```python
from build123d import *

# Parameters (mm, degrees)
F1_DEPTH = 18.1


with BuildPart() as f1:
    # F0 (on Top) → F1 (new body)
    with BuildSketch(Plane.XY):
        with BuildLine():
            ThreePointArc((24.797365, -3.176582), (24.94929, -1.591519), (25, 0))
            ThreePointArc((25, 0), (24.950482, 1.57272), (24.802124, 3.13921))
            ThreePointArc((24.802124, 3.13921), (24.5233, 4.858782), (24.125403, 6.554762))
            ThreePointArc((24.125403, 6.554762), (23.10419, 9.54968), (21.712851, 12.391614))
            ThreePointArc((21.712851, 12.391614), (20.7972, 13.87359), (19.780568, 15.288203))
            ThreePointArc((19.780568, 15.288203), (17.690984, 17.664345), (15.317994, 19.757507))
            ThreePointArc((15.317994, 19.757507), (13.904914, 20.776269), (12.42432, 21.694153))
            ThreePointArc((12.42432, 21.694153), (9.584486, 23.089773), (6.59111, 24.115498))
            ThreePointArc((6.59111, 24.115498), (4.895732, 24.51595), (3.176582, 24.797365))
            ThreePointArc((3.176582, 24.797365), (0.018837, 24.999993), (-3.13921, 24.802124))
            ThreePointArc((-3.13921, 24.802124), (-4.858782, 24.5233), (-6.554762, 24.125403))
            ThreePointArc((-6.554762, 24.125403), (-9.54968, 23.10419), (-12.391614, 21.712851))
            ThreePointArc((-12.391614, 21.712851), (-13.87359, 20.7972), (-15.288203, 19.780568))
            ThreePointArc((-15.288203, 19.780568), (-17.664345, 17.690984), (-19.757507, 15.317994))
            ThreePointArc((-19.757507, 15.317994), (-20.776269, 13.904914), (-21.694153, 12.42432))
            ThreePointArc((-21.694153, 12.42432), (-23.089773, 9.584486), (-24.115498, 6.59111))
            ThreePointArc((-24.115498, 6.59111), (-24.51595, 4.895732), (-24.797365, 3.176582))
            ThreePointArc((-24.797365, 3.176582), (-24.999993, 0.018837), (-24.802124, -3.13921))
            ThreePointArc((-24.802124, -3.13921), (-24.5233, -4.858782), (-24.125403, -6.554762))
            ThreePointArc((-24.125403, -6.554762), (-23.10419, -9.54968), (-21.712851, -12.391614))
            ThreePointArc((-21.712851, -12.391614), (-20.7972, -13.87359), (-19.780568, -15.288203))
            ThreePointArc((-19.780568, -15.288203), (-17.690984, -17.664345), (-15.317994, -19.757507))
            ThreePointArc((-15.317994, -19.757507), (-13.904914, -20.776269), (-12.42432, -21.694153))
            ThreePointArc((-12.42432, -21.694153), (-9.584486, -23.089773), (-6.59111, -24.115498))
            ThreePointArc((-6.59111, -24.115498), (-4.895732, -24.51595), (-3.176582, -24.797365))
            ThreePointArc((-3.176582, -24.797365), (-0.018837, -24.999993), (3.13921, -24.802124))
            ThreePointArc((3.13921, -24.802124), (4.858782, -24.5233), (6.554762, -24.125403))
            ThreePointArc((6.554762, -24.125403), (9.54968, -23.10419), (12.391614, -21.712851))
            ThreePointArc((12.391614, -21.712851), (13.87359, -20.7972), (15.288203, -19.780568))
            ThreePointArc((15.288203, -19.780568), (17.664345, -17.690984), (19.757507, -15.317994))
            ThreePointArc((19.757507, -15.317994), (20.776269, -13.904914), (21.694153, -12.42432))
            ThreePointArc((21.694153, -12.42432), (23.089773, -9.584486), (24.115498, -6.59111))
            ThreePointArc((24.115498, -6.59111), (24.51595, -4.895732), (24.797365, -3.176582))
        make_face()
        with BuildLine():
            ThreePointArc((24.802124, 3.13921), (24.950482, 1.57272), (25, 0))
            ThreePointArc((25, 0), (24.94929, -1.591519), (24.797365, -3.176582))
            Line((24.797365, -3.176582), (28.354543, -2.044125))
            Line((28.354543, -2.044125), (28.354543, 1.937519))
            Line((28.354543, 1.937519), (24.802124, 3.13921))
        make_face()
        with BuildLine():
            ThreePointArc((21.712851, 12.391614), (23.10419, 9.54968), (24.125403, 6.554762))
            Line((24.125403, 6.554762), (26.978435, 8.962289))
            Line((26.978435, 8.962289), (25.454726, 12.640848))
            Line((25.454726, 12.640848), (21.712851, 12.391614))
        make_face()
        with BuildLine():
            Line((26.937638, -9.06078), (24.115498, -6.59111))
            ThreePointArc((24.115498, -6.59111), (23.089773, -9.584486), (21.694153, -12.42432))
            Line((21.694153, -12.42432), (25.413929, -12.739339))
            Line((25.413929, -12.739339), (26.937638, -9.06078))
        make_face()
        with BuildLine():
            ThreePointArc((15.317994, 19.757507), (17.690984, 17.664345), (19.780568, 15.288203))
            Line((19.780568, 15.288203), (21.495104, 18.604275))
            Line((21.495104, 18.604275), (18.679657, 21.419722))
            Line((18.679657, 21.419722), (15.317994, 19.757507))
        make_face()
        with BuildLine():
            Line((21.419722, -18.679657), (19.757507, -15.317994))
            ThreePointArc((19.757507, -15.317994), (17.664345, -17.690984), (15.288203, -19.780568))
            Line((15.288203, -19.780568), (18.604275, -21.495104))
            Line((18.604275, -21.495104), (21.419722, -18.679657))
        make_face()
        with BuildLine():
            ThreePointArc((6.59111, 24.115498), (9.584486, 23.089773), (12.42432, 21.694153))
            Line((12.42432, 21.694153), (12.739339, 25.413929))
            Line((12.739339, 25.413929), (9.06078, 26.937638))
            Line((9.06078, 26.937638), (6.59111, 24.115498))
        make_face()
        with BuildLine():
            Line((12.640848, -25.454726), (12.391614, -21.712851))
            ThreePointArc((12.391614, -21.712851), (9.54968, -23.10419), (6.554762, -24.125403))
            Line((6.554762, -24.125403), (8.962289, -26.978435))
            Line((8.962289, -26.978435), (12.640848, -25.454726))
        make_face()
        with BuildLine():
            ThreePointArc((-3.13921, 24.802124), (0.018837, 24.999993), (3.176582, 24.797365))
            Line((3.176582, 24.797365), (2.044125, 28.354543))
            Line((2.044125, 28.354543), (-1.937519, 28.354543))
            Line((-1.937519, 28.354543), (-3.13921, 24.802124))
        make_face()
        with BuildLine():
            Line((1.937519, -28.354543), (3.13921, -24.802124))
            ThreePointArc((3.13921, -24.802124), (-0.018837, -24.999993), (-3.176582, -24.797365))
            Line((-3.176582, -24.797365), (-2.044125, -28.354543))
            Line((-2.044125, -28.354543), (1.937519, -28.354543))
        make_face()
        with BuildLine():
            ThreePointArc((-12.391614, 21.712851), (-9.54968, 23.10419), (-6.554762, 24.125403))
            Line((-6.554762, 24.125403), (-8.962289, 26.978435))
            Line((-8.962289, 26.978435), (-12.640848, 25.454726))
            Line((-12.640848, 25.454726), (-12.391614, 21.712851))
        make_face()
        with BuildLine():
            Line((-9.06078, -26.937638), (-6.59111, -24.115498))
            ThreePointArc((-6.59111, -24.115498), (-9.584486, -23.089773), (-12.42432, -21.694153))
            Line((-12.42432, -21.694153), (-12.739339, -25.413929))
            Line((-12.739339, -25.413929), (-9.06078, -26.937638))
        make_face()
        with BuildLine():
            ThreePointArc((-19.757507, 15.317994), (-17.664345, 17.690984), (-15.288203, 19.780568))
            Line((-15.288203, 19.780568), (-18.604275, 21.495104))
            Line((-18.604275, 21.495104), (-21.419722, 18.679657))
            Line((-21.419722, 18.679657), (-19.757507, 15.317994))
        make_face()
        with BuildLine():
            Line((-18.679657, -21.419722), (-15.317994, -19.757507))
            ThreePointArc((-15.317994, -19.757507), (-17.690984, -17.664345), (-19.780568, -15.288203))
            Line((-19.780568, -15.288203), (-21.495104, -18.604275))
            Line((-21.495104, -18.604275), (-18.679657, -21.419722))
        make_face()
        with BuildLine():
            ThreePointArc((-24.115498, 6.59111), (-23.089773, 9.584486), (-21.694153, 12.42432))
            Line((-21.694153, 12.42432), (-25.413929, 12.739339))
            Line((-25.413929, 12.739339), (-26.937638, 9.06078))
            Line((-26.937638, 9.06078), (-24.115498, 6.59111))
        make_face()
        with BuildLine():
            Line((-25.454726, -12.640848), (-21.712851, -12.391614))
            ThreePointArc((-21.712851, -12.391614), (-23.10419, -9.54968), (-24.125403, -6.554762))
            Line((-24.125403, -6.554762), (-26.978435, -8.962289))
            Line((-26.978435, -8.962289), (-25.454726, -12.640848))
        make_face()
        with BuildLine():
            ThreePointArc((-24.802124, -3.13921), (-24.999993, 0.018837), (-24.797365, 3.176582))
            Line((-24.797365, 3.176582), (-28.354543, 2.044125))
            Line((-28.354543, 2.044125), (-28.354543, -1.937519))
            Line((-28.354543, -1.937519), (-24.802124, -3.13921))
        make_face()
    extrude(amount=F1_DEPTH)


solid = f1.part
```
Here's how the part is built. I have some questions about the finished solid (model axes, mm). A direction names the side the tool comes from. Give positions to 0.01 mm unless a question says otherwise; leave off trailing zeros. Write each loop counter-clockwise with the first axis right and the second up, starting at its lowest first coordinate (ties: lowest second). Pieces come first, ordered by that corner, then holes. Notation, with made-up numbers: M 57.5,-32 L 66.5,-32 A15 cw 66.5,-13 Z; hole C 22,65 d2. An arc over 180 degrees is marked long. Put each result on its own line as item: value. Start each with the question number.
Item 1: Will these pins go through, and if not, where does the flat tip stop? pin 1 (4 mm diameter, centred on x = 6.5, z = 2, fed in from -Y); pin 2 (3 mm diameter, centred on x = 7.5, z = 11.5, fed in from -Y); pin 3 (10 mm diameter, centred on x = 14.5, z = 13, fed in from -Y).
Item 2: If we section it at B-B, the plane x = 16.5: Write out the boundary of the cut face in (y, z), then the cut area to 3 significant figures.
Item 3: Thinking about a two-plate mould opening in Y: for faces 6 (the flat face through (7.74, -25.53, 8.92)), 7 (the flat face through (28.355, 0, 9)), 8 (the flat face through (12.58, 23.53, 8.92)), which applies, +Y half, -Y half, draft (parallel to the pull), parting line (faces both ways), or undercut?
Item 4: If we section it at A-A, the plane y = 4: Write out the boundary of the cut face in (x, z).
Item 5: On a 3-axis mill with a long thin cutter (end or side, diameter ignored), from which of +Z, -Z, +X, -X, +Y, -Y can I reach the whole of each face in a straight line? I mean faces 1 (the flat face through (26.165, -10.926, 8.923)), 2 (the flat face through (26.6, 2.53, 8.92)), 3 (the flat face through (-23.61, -12.518, 8.923)), 4 (the flat face through (-20.6, 17.02, 8.92)), 5 (the flat face through (-23.53, 12.58, 8.92)). Say none if no direction works.
Item 6: I need wall thicknesses on L1, parallel to X at y = -25, z = 16.5; L2, parallel to X at y = 6.5, z = 10.25. Which ranges of each line are inside material? Lowest first, please. Write a range as from..to.
Values:
1. pin 1: y = -26.43
1. pin 2: y = -26.98
1. pin 3: y = -26.76
2. outline: M -20.41,0 L 20.34,0 L 20.34,18.1 L -20.41,18.1 Z
2. area: 738 mm²
3. face 6: -Y half
3. face 7: draft
3. face 8: undercut
4. outline: M -24.68,0 L 24.68,0 L 24.68,18.1 L -24.68,18.1 Z
5. face 1: +Z, -Z, +X, -Y
5. face 2: +Z, -Z, +X
5. face 3: +Z, -Z, -Y
5. face 4: +Z, -Z, -X
5. face 5: +Z, -Z, +Y
6. L1: -12.7..-7.37, -3.11..3.07, 7.29..12.61
6. L2: -24.14..24.14
